Input: dimensioned drawing with shaded views. Units: mm. Origin: part minimum x, y, z. A direction names the side the tool comes from. Round coordinates to 2 decimals unless told otherwise and drop trailing zeros. Loops run counter-clockwise (first coordinate to the right, second up) from the corner with the lowest first, then second, coordinate; pieces in that order, holes last.
Item 1: Access query for the marked faces 4, 5 and 6. Directions: +Z, -Z, +X, -X, +Y, -Y. A direction counts if a zero-diameter tool reaches every point of the face in a straight line with its end or side. Return the directions, or none.
Item 2: Pull-direction query (X, two-part tool) for the marked faces 1, 2 and 3; classes: released by +X, released by -X, zero draft, split by the parting line, or undercut.
Item 3: Section query A-A on x = 26. Return loops of the section in (y, z), then the cut area to 3 significant figures.
Item 4: Section query D-D on z = 30. Return loops of the section in (x, y).
Item 5: Section query B-B on z = 16. Return loops of the section in (x, y), then the cut area to 3 significant figures.
Item 6: First-contact query: P1, Ø6, axis at y = 4, z = 15.5, coming from the +X side; P2, Ø1.5, axis at x = 21.5, y = 15.5, coming from the -Z side; P3, Ø8, axis at x = 4, y = 18, coming from the +Z side; P4, Ø10, axis at y = 11.5, z = 11.5, coming from the +X side. Flat tips, straight axial feed; report the tip coordinate or a pass-through.
Item 7: Section query C-C on x = 16. Return loops of the section in (y, z).
Item 8: Ray query, L1, parallel to Y at x = 15, z = 24.5; L2, parallel to X at y = 19.45, z = 5; L3, parallel to X at y = 11.5, z = 16. Return the intervals inside material, ascending.
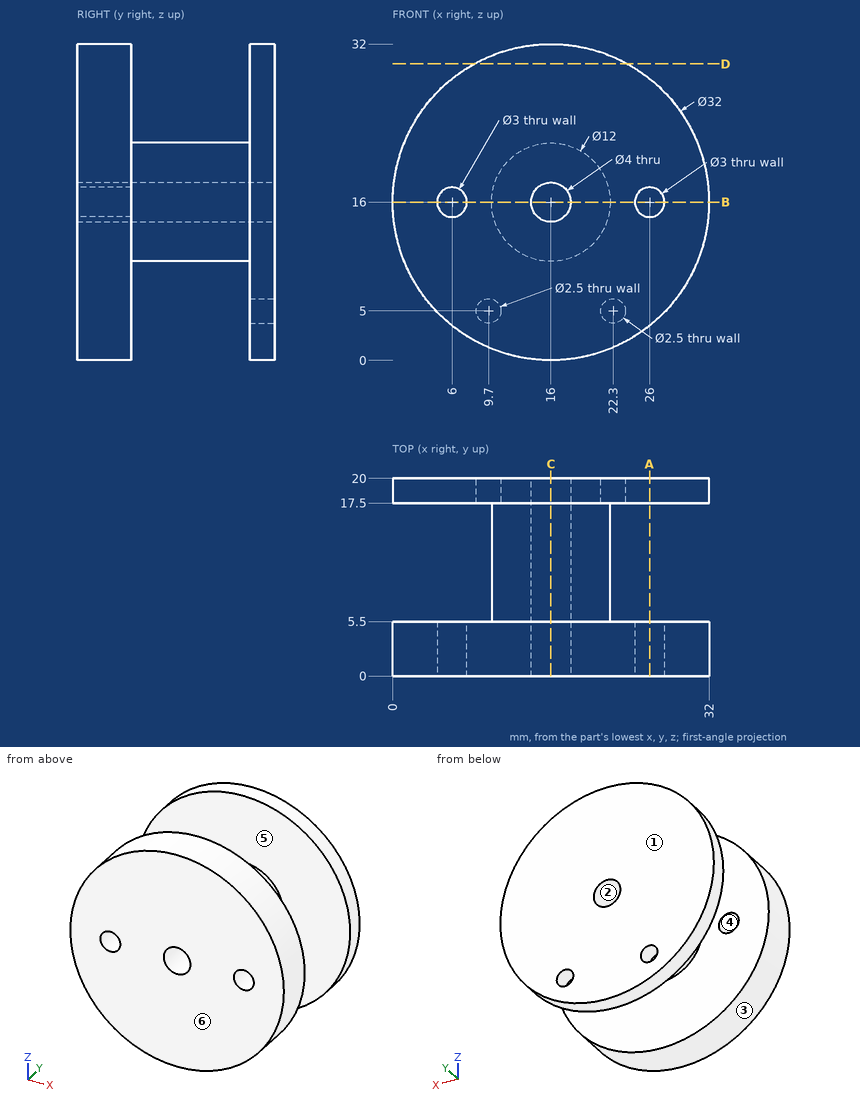
Data:
1. face 4: -Y
1. face 5: none
1. face 6: +Z, -Z, +X, -X, -Y
2. face 1: zero draft
2. face 2: undercut
2. face 3: split by the parting line
3. outline: (0, 3.51) - (5.5, 3.51) - (5.5, 14.5) - (0, 14.5) - close; (0, 17.5) - (5.5, 17.5) - (5.5, 28.49) - (0, 28.49) - close; (17.5, 3.51) - (20, 3.51) - (20, 28.49) - (17.5, 28.49) - close
3. area: 183 mm2
4. outline: (8.25, 0) - (23.75, 0) - (23.75, 5.5) - (8.25, 5.5) - close; (8.25, 17.5) - (23.75, 17.5) - (23.75, 20) - (8.25, 20) - close
5. outline: (0, 0) - (4.5, 0) - (4.5, 5.5) - (0, 5.5) - close; (0, 17.5) - (10, 17.5) - (10, 5.5) - (7.5, 5.5) - (7.5, 0) - (14, 0) - (14, 20) - (0, 20) - close; (18, 0) - (24.5, 0) - (24.5, 5.5) - (22, 5.5) - (22, 17.5) - (32, 17.5) - (32, 20) - (18, 20) - close; (27.5, 0) - (32, 0) - (32, 5.5) - (27.5, 5.5) - close
5. area: 287 mm2
6. P1: stops at x = 32
6. P2: stops at z = 12.33
6. P3: stops at z = 29.86
6. P4: stops at x = 22
7. outline: (0, 0) - (5.5, 0) - (5.5, 10) - (17.5, 10) - (17.5, 0) - (20, 0) - (20, 14) - (0, 14) - close; (0, 18) - (20, 18) - (20, 32) - (17.5, 32) - (17.5, 22) - (5.5, 22) - (5.5, 32) - (0, 32) - close
8. L1: y = 0 to 5.5, 17.5 to 20
8. L2: x = 4.38 to 8.45, 10.95 to 21.05, 23.55 to 27.62
8. L3: x = 10 to 14, 18 to 22
